from build123d import *

# Parameters (mm, degrees)
BASE_FLANGE1_DEPTH             = 104.7
EDGE_FLANGE1_STRIP_W           = 6
EDGE_FLANGE1_STRIP_H           = 1
EDGE_FLANGE1_STRIP_CUT_DEPTH   = 821.4
EDGE_FLANGE1_RELIEF_W          = 6.5
EDGE_FLANGE1_RELIEF_H          = 0.5
EDGE_FLANGE1_RELIEF_CUT_DEPTH  = 1
EDGE_FLANGE1_DEPTH             = 821.4
EDGE_FLANGE2_STRIP_W           = 6
EDGE_FLANGE2_STRIP_H           = 1
EDGE_FLANGE2_STRIP_CUT_DEPTH   = 821.4
EDGE_FLANGE2_DEPTH             = 821.4
EDGE_FLANGE3_STRIP_W           = 6
EDGE_FLANGE3_STRIP_H           = 1
EDGE_FLANGE3_STRIP_CUT_DEPTH   = 80
EDGE_FLANGE3_RELIEF_W          = 6.5
EDGE_FLANGE3_RELIEF_H          = 0.5
EDGE_FLANGE3_RELIEF_CUT_DEPTH  = 1
EDGE_FLANGE3_DEPTH             = 80
EDGE_FLANGE4_STRIP_W           = 6
EDGE_FLANGE4_STRIP_H           = 1
EDGE_FLANGE4_STRIP_CUT_DEPTH   = 80
EDGE_FLANGE4_DEPTH             = 80
EDGE_FLANGE5_STRIP_W           = 6
EDGE_FLANGE5_STRIP_H           = 1
EDGE_FLANGE5_STRIP_CUT_DEPTH   = 777.4
EDGE_FLANGE5_RELIEF_W          = 6.5
EDGE_FLANGE5_RELIEF_H          = 0.5
EDGE_FLANGE5_RELIEF_CUT_DEPTH  = 1
EDGE_FLANGE5_DEPTH             = 777.4
SKETCH25_R                     = 2.5
CUT_EXTRUDE1_DEPTH             = 3
SKETCH26_R                     = 2.5
CUT_EXTRUDE2_DEPTH             = 3
CUT_EXTRUDE2_DIRECTION_2_REACH = 857.86
EDGE_FLANGE7_STRIP_W           = 6
EDGE_FLANGE7_STRIP_H           = 1
EDGE_FLANGE7_STRIP_CUT_DEPTH   = 777.4
EDGE_FLANGE7_DEPTH             = 777.4
EDGE_FLANGE7_FLAT_DEPTH        = 1
SKETCH30_W                     = 21
SKETCH30_H                     = 65.6
CUT_EXTRUDE3_DEPTH             = 10
FILLET1_R                      = 2


# Sheet-metal steps are written as plain solids
with BuildPart() as part:
    # Sketch1 → Base-Flange1 (new body)
    with BuildSketch(Plane.XY):
        with BuildLine():
            Line((-430.7, -100), (-430.7, -15))
            ThreePointArc((-430.7, -15), (-426.306601718, -4.393398282), (-415.7, 0))
            Line((-415.7, 0), (415.7, 0))
            ThreePointArc((415.7, 0), (426.306601718, -4.393398282), (430.7, -15))
            Line((430.7, -15), (430.7, -100))
            Line((430.7, -100), (431.7, -100))
            Line((431.7, -100), (431.7, -15))
            ThreePointArc((431.7, -15), (427.013708499, -3.686291501), (415.7, 1))
            Line((415.7, 1), (-415.7, 1))
            ThreePointArc((-415.7, 1), (-427.013708499, -3.686291501), (-431.7, -15))
            Line((-431.7, -15), (-431.7, -100))
            Line((-431.7, -100), (-430.7, -100))
        make_face()
    extrude(amount=BASE_FLANGE1_DEPTH)

    # Edge-Flange1 strip (across the edge) → Edge-Flange1 strip cut (cut)
    with BuildSketch(Plane(origin=(-410.7, 0, 0), x_dir=(0, 0, 1), z_dir=(1, 0, 0))):
        with Locations((-2, -0.5)):
            Rectangle(EDGE_FLANGE1_STRIP_W, EDGE_FLANGE1_STRIP_H)
    extrude(amount=EDGE_FLANGE1_STRIP_CUT_DEPTH, mode=Mode.SUBTRACT)

    # Edge-Flange1 relief (on the sheet) → Edge-Flange1 relief cut (cut)
    with BuildSketch(Plane(origin=(-410.7, 0, 1), x_dir=(0, 0, 1), z_dir=(0, -1, 0))):
        with Locations((-2.75, 0.25)):
            Rectangle(EDGE_FLANGE1_RELIEF_W, EDGE_FLANGE1_RELIEF_H)
        with Locations((-2.75, -821.65)):
            Rectangle(EDGE_FLANGE1_RELIEF_W, EDGE_FLANGE1_RELIEF_H)
    extrude(amount=-EDGE_FLANGE1_RELIEF_CUT_DEPTH, mode=Mode.SUBTRACT)

    # Edge-Flange1 section (across the edge) → Edge-Flange1 (add)
    with BuildSketch(Plane(origin=(-410.7, 0, 0), x_dir=(0, 0, 1), z_dir=(1, 0, 0))):
        with BuildLine():
            Line((-1, 1), (-1, 19))
            Line((-1, 19), (0, 19))
            Line((0, 19), (0, 1))
            ThreePointArc((0, 1), (0.292893219, 0.292893219), (1, 0))
            Line((1, 0), (1, -1))
            ThreePointArc((1, -1), (-0.414213562, -0.414213562), (-1, 1))
        make_face()
    extrude(amount=EDGE_FLANGE1_DEPTH)

    # Edge-Flange2 strip (across the edge) → Edge-Flange2 strip cut (cut)
    with BuildSketch(Plane(origin=(-410.7, -19, 0), x_dir=(0, 1, 0), z_dir=(1, 0, 0))):
        with Locations((-1, -0.5)):
            Rectangle(EDGE_FLANGE2_STRIP_W, EDGE_FLANGE2_STRIP_H)
    extrude(amount=EDGE_FLANGE2_STRIP_CUT_DEPTH, mode=Mode.SUBTRACT)

    # Edge-Flange2 section (across the edge) → Edge-Flange2 (add)
    with BuildSketch(Plane(origin=(-410.7, -19, 0), x_dir=(0, 1, 0), z_dir=(1, 0, 0))):
        with BuildLine():
            Line((0, 1), (0, 12))
            Line((0, 12), (1, 12))
            Line((1, 12), (1, 1))
            ThreePointArc((1, 1), (1.292893219, 0.292893219), (2, 0))
            Line((2, 0), (2, -1))
            ThreePointArc((2, -1), (0.585786438, -0.414213562), (0, 1))
        make_face()
    extrude(amount=EDGE_FLANGE2_DEPTH)

    # Edge-Flange3 strip (across the edge) → Edge-Flange3 strip cut (cut)
    with BuildSketch(Plane(origin=(-430.7, -100, 0), x_dir=(0, 0, 1), z_dir=(0, 1, 0))):
        with Locations((-2, -0.5)):
            Rectangle(EDGE_FLANGE3_STRIP_W, EDGE_FLANGE3_STRIP_H)
    edge_flange3_strip_cut = extrude(amount=EDGE_FLANGE3_STRIP_CUT_DEPTH, mode=Mode.SUBTRACT)

    # Edge-Flange3 relief (on the sheet) → Edge-Flange3 relief cut (cut)
    with BuildSketch(Plane(origin=(-430.7, -100, 1), x_dir=(0, 0, 1), z_dir=(1, 0, 0))):
        with Locations((-2.75, -80.25)):
            Rectangle(EDGE_FLANGE3_RELIEF_W, EDGE_FLANGE3_RELIEF_H)
    edge_flange3_relief_cut = extrude(amount=-EDGE_FLANGE3_RELIEF_CUT_DEPTH, mode=Mode.SUBTRACT)

    # Edge-Flange3 section (across the edge) → Edge-Flange3 (add)
    with BuildSketch(Plane(origin=(-430.7, -100, 0), x_dir=(0, 0, 1), z_dir=(0, 1, 0))):
        with BuildLine():
            Line((-1, 1), (-1, 19))
            Line((-1, 19), (0, 19))
            Line((0, 19), (0, 1))
            ThreePointArc((0, 1), (0.292893219, 0.292893219), (1, 0))
            Line((1, 0), (1, -1))
            ThreePointArc((1, -1), (-0.414213562, -0.414213562), (-1, 1))
        make_face()
    edge_flange3 = extrude(amount=EDGE_FLANGE3_DEPTH)

    # Edge-Flange4 strip (across the edge) → Edge-Flange4 strip cut (cut)
    with BuildSketch(Plane(origin=(-411.7, -100, 0), x_dir=(-1, 0, 0), z_dir=(0, 1, 0))):
        with Locations((-1, -0.5)):
            Rectangle(EDGE_FLANGE4_STRIP_W, EDGE_FLANGE4_STRIP_H)
    edge_flange4_strip_cut = extrude(amount=EDGE_FLANGE4_STRIP_CUT_DEPTH, mode=Mode.SUBTRACT)

    # Edge-Flange4 section (across the edge) → Edge-Flange4 (add)
    with BuildSketch(Plane(origin=(-411.7, -100, 0), x_dir=(-1, 0, 0), z_dir=(0, 1, 0))):
        with BuildLine():
            Line((0, 1), (0, 12))
            Line((0, 12), (1, 12))
            Line((1, 12), (1, 1))
            ThreePointArc((1, 1), (1.292893219, 0.292893219), (2, 0))
            Line((2, 0), (2, -1))
            ThreePointArc((2, -1), (0.585786438, -0.414213562), (0, 1))
        make_face()
    edge_flange4 = extrude(amount=EDGE_FLANGE4_DEPTH)

    # Mirror1: Edge-Flange3 strip cut, Edge-Flange3 relief cut, Edge-Flange3, Edge-Flange4 strip cut, Edge-Flange4 across plane
    add(edge_flange3_strip_cut.mirror(Plane(origin=(0, 0, 0), x_dir=(0, 0, 1), z_dir=(1, 0, 0))), mode=Mode.SUBTRACT)
    add(edge_flange3_relief_cut.mirror(Plane(origin=(0, 0, 0), x_dir=(0, 0, 1), z_dir=(1, 0, 0))), mode=Mode.SUBTRACT)
    add(edge_flange3.mirror(Plane(origin=(0, 0, 0), x_dir=(0, 0, 1), z_dir=(1, 0, 0))))
    add(edge_flange4_strip_cut.mirror(Plane(origin=(0, 0, 0), x_dir=(0, 0, 1), z_dir=(1, 0, 0))), mode=Mode.SUBTRACT)
    add(edge_flange4.mirror(Plane(origin=(0, 0, 0), x_dir=(0, 0, 1), z_dir=(1, 0, 0))))

    # Edge-Flange5 strip (across the edge) → Edge-Flange5 strip cut (cut)
    with BuildSketch(Plane(origin=(388.7, 0, 104.7), x_dir=(0, 0, -1), z_dir=(-1, 0, 0))):
        with Locations((-2, -0.5)):
            Rectangle(EDGE_FLANGE5_STRIP_W, EDGE_FLANGE5_STRIP_H)
    extrude(amount=EDGE_FLANGE5_STRIP_CUT_DEPTH, mode=Mode.SUBTRACT)

    # Edge-Flange5 relief (on the sheet) → Edge-Flange5 relief cut (cut)
    with BuildSketch(Plane(origin=(388.7, 0, 103.7), x_dir=(0, 0, -1), z_dir=(0, -1, 0))):
        with Locations((-2.75, 0.25)):
            Rectangle(EDGE_FLANGE5_RELIEF_W, EDGE_FLANGE5_RELIEF_H)
        with Locations((-2.75, -777.65)):
            Rectangle(EDGE_FLANGE5_RELIEF_W, EDGE_FLANGE5_RELIEF_H)
    extrude(amount=-EDGE_FLANGE5_RELIEF_CUT_DEPTH, mode=Mode.SUBTRACT)

    # Edge-Flange5 section (across the edge) → Edge-Flange5 (add)
    with BuildSketch(Plane(origin=(388.7, 0, 104.7), x_dir=(0, 0, -1), z_dir=(-1, 0, 0))):
        with BuildLine():
            Line((-1, 1), (-1, 35.5))
            Line((-1, 35.5), (0, 35.5))
            Line((0, 35.5), (0, 1))
            ThreePointArc((0, 1), (0.292893219, 0.292893219), (1, 0))
            Line((1, 0), (1, -1))
            ThreePointArc((1, -1), (-0.414213562, -0.414213562), (-1, 1))
        make_face()
    extrude(amount=EDGE_FLANGE5_DEPTH)

    # Sketch25 → Cut-Extrude1 (cut)
    with BuildSketch(Plane.XZ.offset(19)):
        with Locations(Location((-349.7, 6, 0), (0, 0, 270))):
            Circle(SKETCH25_R)
        with Locations(Location((-169.7, 6, 0), (0, 0, 270))):
            Circle(SKETCH25_R)
        with Locations(Location((10.3, 6, 0), (0, 0, 270))):
            Circle(SKETCH25_R)
        with Locations(Location((190.3, 6, 0), (0, 0, 270))):
            Circle(SKETCH25_R)
        with Locations(Location((370.3, 6, 0), (0, 0, 270))):
            Circle(SKETCH25_R)
        with Locations((550.3, 6)):
            Circle(SKETCH25_R)
        with Locations((730.3, 6)):
            Circle(SKETCH25_R)
    extrude(amount=-CUT_EXTRUDE1_DEPTH, mode=Mode.SUBTRACT)

    # Sketch26 → Cut-Extrude2 (cut)
    with BuildSketch(Plane(origin=(-411.7, 0, 0), x_dir=(0, 0, -1), z_dir=(1, 0, 0))):
        with Locations((-6, -68)):
            Circle(SKETCH26_R)
    extrude(amount=-CUT_EXTRUDE2_DEPTH, mode=Mode.SUBTRACT)

    # Cut-Extrude2 direction 2: up to this face of the body (flat: up to its plane)
    cut_extrude2_direction_2_end = Plane(part.part.faces().sort_by_distance((412.7, -60, 6.5))[0])
    # Sketch26 → Cut-Extrude2 direction 2 (cut, up to the picked face)
    with BuildSketch(Plane(origin=(-411.7, 0, 0), x_dir=(0, 0, -1), z_dir=(1, 0, 0)), mode=Mode.PRIVATE) as cut_extrude2_direction_2_sk1:
        with Locations((-6, -68)):
            Circle(SKETCH26_R)
    cut_extrude2_direction_2_tool1 = split(extrude(cut_extrude2_direction_2_sk1.sketch, amount=CUT_EXTRUDE2_DIRECTION_2_REACH, mode=Mode.PRIVATE), bisect_by=cut_extrude2_direction_2_end, keep=Keep.BOTH, mode=Mode.PRIVATE)
    add(cut_extrude2_direction_2_tool1.solids().sort_by(Axis((-411.7, -68, 6), (1, 0, 0)))[0], mode=Mode.SUBTRACT)

    # Edge-Flange7 strip (across the edge) → Edge-Flange7 strip cut (cut)
    with BuildSketch(Plane(origin=(388.7, -35.5, 104.7), x_dir=(0, 1, 0), z_dir=(-1, 0, 0))):
        with Locations((-1, -0.5)):
            Rectangle(EDGE_FLANGE7_STRIP_W, EDGE_FLANGE7_STRIP_H)
    extrude(amount=EDGE_FLANGE7_STRIP_CUT_DEPTH, mode=Mode.SUBTRACT)

    # Edge-Flange7 bend section (across the edge) → Edge-Flange7 (add)
    with BuildSketch(Plane(origin=(388.7, -35.5, 104.7), x_dir=(0, 1, 0), z_dir=(-1, 0, 0))):
        with BuildLine():
            Line((0, 1), (1, 1))
            ThreePointArc((1, 1), (1.292893219, 0.292893219), (2, 0))
            Line((2, 0), (2, -1))
            ThreePointArc((2, -1), (0.585786438, -0.414213562), (0, 1))
        make_face()
    extrude(amount=EDGE_FLANGE7_DEPTH)

    # Edge-Flange7 profile (on flange) → Edge-Flange7 flat (add)
    with BuildSketch(Plane(origin=(0, -35.5, 104.7), x_dir=(1, 0, 0), z_dir=(0, 1, 0))):
        with BuildLine():
            Line((-388.7, 1), (388.7, 1))
            Line((388.7, 1), (388.7, 28))
            ThreePointArc((388.7, 28), (387.821320344, 30.121320344), (385.7, 31))
            Line((385.7, 31), (-385.7, 31))
            ThreePointArc((-385.7, 31), (-387.821320344, 30.121320344), (-388.7, 28))
            Line((-388.7, 28), (-388.7, 1))
        make_face()
    extrude(amount=EDGE_FLANGE7_FLAT_DEPTH)

    # Sketch30 → Cut-Extrude3 (cut)
    with BuildSketch(Plane(origin=(431.7, 0, 0), x_dir=(0, 0, -1), z_dir=(1, 0, 0))):
        with Locations((-94.2, -67.2)):
            Rectangle(SKETCH30_W, SKETCH30_H)
    extrude(amount=-CUT_EXTRUDE3_DEPTH, mode=Mode.SUBTRACT)

    # Fillet1
    fillet1_edges = [part.edges().sort_by_distance(p)[0] for p in [
        (431.2, -34.4, 104.7),
    ]]
    fillet(fillet1_edges, radius=FILLET1_R)


solid = part.part
Read the model definition and answer for the solid it produces. Units are mm, in the model's axes. A direction names the side the tool comes from. Coordinates: 2 decimals unless noted, no trailing zeros. Order: outer loops, then holes, each group sorted by start corner. A loop starts at its lowest first (then second) coordinate and runs counter-clockwise, first axis right, second up. Notation, with made-up numbers: (48.25, 26.5) - (101.25, 26.5) arc R37 ccw to (101.25, 63.5) - close; hole circle Ø2 at (-19, 39). An arc over 180 degrees is marked (long way). Use one line per item in the form item = value.
(1) Section D-D, the plane z = 50.5 is taken. Give the vertices of the cut face in (x, y).
Computed values:
outline = (-431.7, -100) - (-430.7, -100) - (-430.7, -15) arc R15 cw to (-415.7, 0) - (415.7, 0) arc R15 cw to (430.7, -15) - (430.7, -100) - (431.7, -100) - (431.7, -15) arc R16 ccw to (415.7, 1) - (-415.7, 1) arc R16 ccw to (-431.7, -15) - close
(2) Straight lines are drawn through the part: L1, parallel to Y at x = 412, z = 6; L2, parallel to X at y = -83, z = 43.5; L3, parallel to Y at x = 29.5, z = 97. For each, find the intervals that lie inside material, in ascending order.
Computed values:
L1 = -100 to -70.5, -65.5 to -20, 0 to 1
L2 = -431.7 to -430.7, 430.7 to 431.7
L3 = -35.5 to -34.5, 0 to 1
(3) Section C-C, the plane x = 211 is taken. Give the vertices of the cut face in (y, z).
Computed values:
outline = (-35.5, 73.7) - (-34.5, 73.7) - (-34.5, 103.7) arc R1 cw to (-33.5, 104.7) - (-1, 104.7) arc R1 cw to (0, 103.7) - (0, 1) arc R1 cw to (-1, 0) - (-17, 0) arc R1 cw to (-18, 1) - (-18, 12) - (-19, 12) - (-19, 1) arc R2 ccw to (-17, -1) - (-1, -1) arc R2 ccw to (1, 1) - (1, 103.7) arc R2 ccw to (-1, 105.7) - (-33.5, 105.7) arc R2 ccw to (-35.5, 103.7) - close
(4) For a pull along Z with two mould halves and no side action, classify faces 1 (the face through (-6, 0, 52)), 2 (the face through (-431, -49, 104.7)), 3 (the face through (-426.42, -4.51, 51.62)), 4 (the face through (422, -61, -1)) as pulls with the +Z half, pulls with the -Z half, needs draft (parallel to the pull), parting line crosses it, or undercut.
Computed values:
face_1 = undercut
face_2 = pulls with the +Z half
face_3 = needs draft
face_4 = pulls with the -Z half
(5) Which of the six approach directions +Z, -Z, +X, -X, +Y, -Y give full straight-line access (tool end or side, diameter ignored) to faces 5 (the face through (-5, -35.5, 88)), 6 (the face through (-5, -34.5, 88)), 7 (the face through (430.7, -57, 40))?
Computed values:
face_5 = +Z, -Z, -Y
face_6 = -Z
face_7 = +Z, -Y
(6) Given pin 1 Ø3 at (x, z) = (108, 66.5) entering from -Y; pin 2 Ø14.5 at (x, z) = (425.5, 4) entering from +Y; pin 3 Ø3.5 at (x, z) = (-185, 7) entering from -Y, each flat-ended and moving along its own axis, determine where each tip first touches the part or whether it passes through.
Computed values:
pin_1 = 0
pin_2 = 0.8
pin_3 = -19
(7) Section A-A, the plane y = -56.5 is taken. Give the vertices of the cut face in (x, z), then the cut area to 3 significant figures.
Computed values:
outline = (-431.7, 1) arc R2 ccw to (-429.7, -1) - (-413.7, -1) arc R2 ccw to (-411.7, 1) - (-411.7, 12) - (-412.7, 12) - (-412.7, 1) arc R1 cw to (-413.7, 0) - (-429.7, 0) arc R1 cw to (-430.7, 1) - (-430.7, 104.7) - (-431.7, 104.7) - close; (411.7, 1) arc R2 ccw to (413.7, -1) - (429.7, -1) arc R2 ccw to (431.7, 1) - (431.7, 83.7) - (430.7, 83.7) - (430.7, 1) arc R1 cw to (429.7, 0) - (413.7, 0) arc R1 cw to (412.7, 1) - (412.7, 12) - (411.7, 12) - close
area = 250 mm²
(8) Section B-B, the plane z = 95 is taken. Give the vertices of the cut face in (x, y).
Computed values:
outline = (-431.7, -100) - (-430.7, -100) - (-430.7, -15) arc R15 cw to (-415.7, 0) - (415.7, 0) arc R15 cw to (430.7, -15) - (430.7, -34.4) - (431.7, -34.4) - (431.7, -15) arc R16 ccw to (415.7, 1) - (-415.7, 1) arc R16 ccw to (-431.7, -15) - close; (-388.7, -35.5) - (388.7, -35.5) - (388.7, -34.5) - (-388.7, -34.5) - close
